CAD build for the part. Positions are in the model's coordinates, mm. A direction names the side the tool comes from. Coordinates: 2 decimals unless noted, no trailing zeros. Loops run counter-clockwise (first coordinate to the right, second up) from the corner with the lowest first, then second, coordinate; pieces in that order, holes last. Notation, with made-up numbers: M -39,29.5 L -16,29.5 A13 cw -16,48.5 Z; hole C 33.5,82 d7. An arc over 180 degrees is marked long. Answer as a JSON object with one key per item and string values. Group by question number.
```python
from build123d import *

# Parameters (mm, degrees)
SKETCH_1_W          = 100
SKETCH_1_H          = 100
EXTRUDE_1_DEPTH     = 10
SKETCH_2_R          = 5
CUT_EXTRUDE_1_DEPTH = 7
SKETCH_3_R          = 1.5
CUT_EXTRUDE_2_DEPTH = 142.774468788
SKETCH_4_R          = 4.5
CUT_EXTRUDE_3_DEPTH = 142.774468788
SKETCH_5_R          = 6.5
CUT_EXTRUDE_4_DEPTH = 3
SKETCH_6_R          = 1.5
CUT_EXTRUDE_5_DEPTH = 142.774468788
SKETCH_7_R          = 1.4
CUT_EXTRUDE_6_DEPTH = 5


with BuildPart() as part:
    # 草图1 → 凸台-拉伸1 (new body)
    with BuildSketch(Plane(origin=(0, 0, 0), x_dir=(1, 0, 0), z_dir=(0, 1, 0))):
        with Locations((50, -50)):
            Rectangle(SKETCH_1_W, SKETCH_1_H)
    extrude(amount=EXTRUDE_1_DEPTH)

    # 草图2 → 切除-拉伸1 (cut)
    with BuildSketch(Plane(origin=(0, 10, 0), x_dir=(1, 0, 0), z_dir=(0, 1, 0))):
        with Locations(Location((10, -10, 0), (0, 0, 270))):
            Circle(SKETCH_2_R)
        with Locations(Location((90, -10, 0), (0, 0, 270))):
            Circle(SKETCH_2_R)
        with Locations(Location((10, -90, 0), (0, 0, 270))):
            Circle(SKETCH_2_R)
        with Locations(Location((90, -90, 0), (0, 0, 270))):
            Circle(SKETCH_2_R)
    extrude(amount=-CUT_EXTRUDE_1_DEPTH, mode=Mode.SUBTRACT)

    # 草图3 → 切除-拉伸2 (cut, through all)
    with BuildSketch(Plane(origin=(0, 10, 0), x_dir=(1, 0, 0), z_dir=(0, 1, 0))):
        with Locations(Location((50, -95, 0), (0, 0, 270))):
            Circle(SKETCH_3_R)
        with Locations(Location((90.414518843, -25, 0), (0, 0, 270))):
            Circle(SKETCH_3_R)
        with Locations(Location((9.585481157, -25, 0), (0, 0, 270))):
            Circle(SKETCH_3_R)
    extrude(amount=-CUT_EXTRUDE_2_DEPTH, mode=Mode.SUBTRACT)

    # 草图4 → 切除-拉伸3 (cut, through all)
    with BuildSketch(Plane(origin=(0, 10, 0), x_dir=(1, 0, 0), z_dir=(0, 1, 0))):
        with Locations(Location((50, -27, 0), (0, 0, 270))):
            Circle(SKETCH_4_R)
    extrude(amount=-CUT_EXTRUDE_3_DEPTH, mode=Mode.SUBTRACT)

    # 草图5 → 切除-拉伸4 (cut)
    with BuildSketch(Plane(origin=(0, 0, 0), x_dir=(-1, 0, 0), z_dir=(0, -1, 0))):
        with Locations(Location((-50, -27, 0), (0, 0, 90))):
            Circle(SKETCH_5_R)
    extrude(amount=-CUT_EXTRUDE_4_DEPTH, mode=Mode.SUBTRACT)

    # 草图6 → 切除-拉伸5 (cut, through all)
    with BuildSketch(Plane(origin=(0, 10, 0), x_dir=(1, 0, 0), z_dir=(0, 1, 0))):
        with Locations(Location((40.56, -59.76, 0), (0, 0, 270))):
            Circle(SKETCH_6_R)
        with Locations(Location((40.56, -75, 0), (0, 0, 270))):
            Circle(SKETCH_6_R)
        with Locations(Location((5, -59.76, 0), (0, 0, 270))):
            Circle(SKETCH_6_R)
        with Locations(Location((5, -75, 0), (0, 0, 270))):
            Circle(SKETCH_6_R)
    extrude(amount=-CUT_EXTRUDE_5_DEPTH, mode=Mode.SUBTRACT)

    # 草图7 → 切除-拉伸6 (cut)
    with BuildSketch(Plane(origin=(0, 0, 0), x_dir=(-1, 0, 0), z_dir=(0, -1, 0))):
        with Locations(Location((-65, -27, 0), (0, 0, 90))):
            Circle(SKETCH_7_R)
        with Locations(Location((-35, -27, 0), (0, 0, 90))):
            Circle(SKETCH_7_R)
    extrude(amount=-CUT_EXTRUDE_6_DEPTH, mode=Mode.SUBTRACT)


solid = part.part
```
Item 1: Slice it at C-C, the plane z = 13. Write the cut outline in (x, y).
Item 2: Slice it at B-B, the plane z = 75. Write the cut outline in (x, y).
Item 3: Pull direction X, two halves, no side cores. Call faces 4 (the flat face through (49, 5, 100)), 5 (the cylindrical face through (64.15, 2.46, 28.11)), 6 (the flat face through (0, 5, 51)): released by +X, released by -X, zero draft, split by the parting line, or undercut.
Item 4: Slice it at A-A, the plane x = 40.56. Write the cut outline in (y, z), then the cut area to 3 significant figures.
Item 5: Slice it at D-D, the plane y = 7.25. Count the separate pieces of the cut face and the enclosed holes in it, then the cut area to 3 significant figures.
Item 6: Drill centre lines: L1, parallel to X at y = 5.5, z = 10; L2, parallel to X at y = 3.35, z = 27; L3, parallel to Z at x = 40, y = 7.75. Where is each one in solid material? Low to high. Write a range as from..to.
Item 7: Pin check, flat tips, straight feed: pin 1 (2 mm diameter, centred on x = 65, z = 27, fed in from -Y); pin 2 (5 mm diameter, centred on x = 10, z = 92, fed in from +Y); pin 3 (5 mm diameter, centred on x = 5, z = 75, fed in from +Y); pin 4 (10.5 mm diameter, centred on x = 50, z = 27, fed in from -Y). Stop position of each tip, or through.
Item 8: Tool access for faces 1 (the cylindrical face through (11.5, 6.55, 14.77)), 2 (the cylindrical face through (48.67, 5.07, 95.69)), 3 (the cylindrical face through (46.045, 1.479, 32.158)): list every direction of +Z, -Z, +X, -X, +Y, -Y with a clear straight run to the whole face (end or side of a thin tool).
Computed:
{
 "1": {"outline": "M 0,0 L 100,0 L 100,10 L 94,10 L 94,3 L 86,3 L 86,10 L 14,10 L 14,3 L 6,3 L 6,10 L 0,10 Z"},
 "2": {"outline": "M 0,0 L 3.5,0 L 3.5,10 L 0,10 Z; M 6.5,0 L 39.06,0 L 39.06,10 L 6.5,10 Z; M 42.06,0 L 100,0 L 100,10 L 42.06,10 Z"},
 "3": {"face 4": "zero draft", "face 5": "undercut", "face 6": "released by -X"},
 "4": {"outline": "M 0,0 L 10,0 L 10,58.26 L 0,58.26 Z; M 0,61.26 L 10,61.26 L 10,73.5 L 0,73.5 Z; M 0,76.5 L 10,76.5 L 10,100 L 0,100 Z", "area": "940 mm2"},
 "5": {"separate pieces": "1", "enclosed holes": "12", "area": "9,570 mm2"},
 "6": {"L1": "0..5, 15..85, 95..100", "L2": "0..33.6, 36.4..45.5, 54.5..63.6, 66.4..100", "L3": "0..58.37, 61.15..73.61, 76.39..100"},
 "7": {"pin 1": "y = 5", "pin 2": "y = 3", "pin 3": "y = 10", "pin 4": "y = 3"},
 "8": {"face 1": "+Y", "face 2": "+Y, -Y", "face 3": "-Y"}
}
